The listing builds one solid part. Answer for the finished solid, in the listing's coordinates (mm). A direction names the side the tool comes from. Coordinates: 2 decimals unless noted, no trailing zeros. Write each loop counter-clockwise with the first axis right and the second up, starting at its lowest first coordinate (ties: lowest second). Pieces come first, ordered by that corner, then holes. Notation, with made-up numbers: M 28,30.25 L 83,30.25 A31 cw 83,62.25 Z; hole C 57,40.25 d4. An arc over 180 degrees is marked long. Answer as a JSON object with one key per item and string values. Group by question number.
from build123d import *

# Parameters (mm, degrees)
SKETCH2_W           = 5
SKETCH2_H           = 7.5
BOSS_EXTRUDE2_DEPTH = 12.5
SKETCH1_W           = 4.5
SKETCH1_H           = 10
BOSS_EXTRUDE4_DEPTH = 37.5


with BuildPart() as part:
    # Sketch2 → Boss-Extrude2 (new body)
    with BuildSketch(Plane.XY.offset(37.5)):
        with Locations((0, 1.25)):
            Rectangle(SKETCH2_W, SKETCH2_H)
    extrude(amount=BOSS_EXTRUDE2_DEPTH)

    # Sketch1 → Boss-Extrude4 (add)
    with BuildSketch(Plane.XY):
        Rectangle(SKETCH1_W, SKETCH1_H)
    extrude(amount=BOSS_EXTRUDE4_DEPTH)


solid = part.part
Item 1: Consider L1, parallel to X at y = -4.5, z = 37; L2, parallel to Y at x = -0.6, z = 45.5; L3, parallel to Z at x = 0.45, y = -4. Determine where each line is inside the solid, lowest interval first. Write a range as from..to.
Item 2: A cutting plane is placed at A-A, the plane y = 4. Write down the section's boundary in (x, z).
Item 3: A cutting plane is placed at B-B, the plane x = 0.45. Write down the section's boundary in (y, z), and give its area (3 significant figures).
Item 4: A cutting plane is placed at C-C, the plane z = 39.5. Write down the section's boundary in (x, y), and give its area (3 significant figures).
Item 5: A cutting plane is placed at D-D, the plane y = -4. Write down the section's boundary in (x, z), and give its area (3 significant figures).
Item 6: Flat-ended cylindrical pins translate along their axes: pin 1 Ø5 at (y, z) = (0, 21.5) entering from +X; pin 2 Ø3 at (x, y) = (0, -4.5) entering from +Z. Find the tip coordinate at first contact, or state that the pin passes through.
Item 7: A tool of negligible diameter and unlimited length cuts with its end or side. For faces 1 (the face through (0, -2.5, 44)), 2 (the face through (0, 5, 25)), 3 (the face through (2.25, 0, 18)), 4 (the face through (-2.25, 0, 18)), from which of +Z, -Z, +X, -X, +Y, -Y can it reach the whole face along a straight path? Write none if from no direction.
Answer:
{
 "1": {"L1": "-2.25..2.25", "L2": "-2.5..5", "L3": "0..37.5"},
 "2": {"outline": "M -2.5,37.5 L -2.25,37.5 L -2.25,0 L 2.25,0 L 2.25,37.5 L 2.5,37.5 L 2.5,50 L -2.5,50 Z"},
 "3": {"outline": "M -5,0 L 5,0 L 5,50 L -2.5,50 L -2.5,37.5 L -5,37.5 Z", "area": "469 mm2"},
 "4": {"outline": "M -2.5,-2.5 L 2.5,-2.5 L 2.5,5 L -2.5,5 Z", "area": "37.5 mm2"},
 "5": {"outline": "M -2.25,0 L 2.25,0 L 2.25,37.5 L -2.25,37.5 Z", "area": "169 mm2"},
 "6": {"pin 1": "x = 2.25", "pin 2": "z = 37.5"},
 "7": {"face 1": "+Z, +X, -X, -Y", "face 2": "+Z, -Z, +X, -X, +Y", "face 3": "-Z, +X, +Y, -Y", "face 4": "-Z, -X, +Y, -Y"}
}
